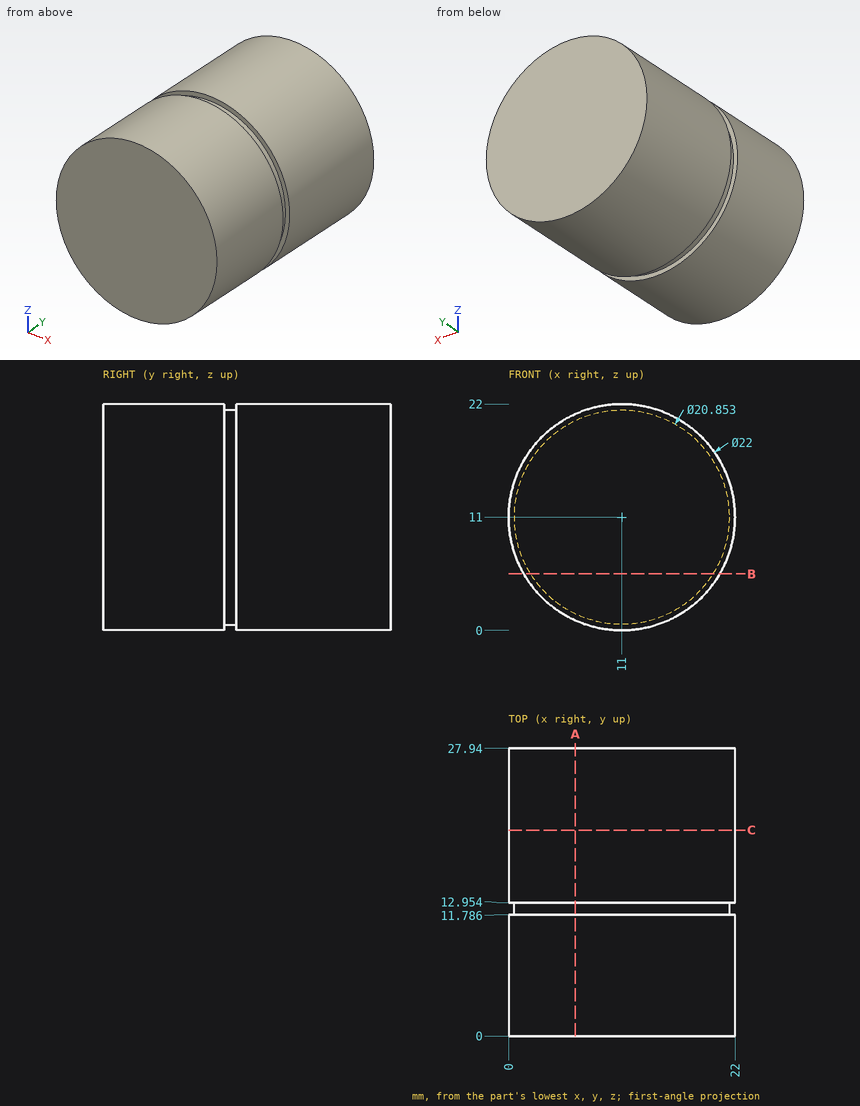
Design review of the part shown in the three views and the two pictorial views. Dimensions are in mm from the part's minimum x, y and z. Give positions to 0.01 mm unless a question says otherwise; leave off trailing zeros. Loops run counter-clockwise (first coordinate to the right, second up) from the corner with the lowest first, then second, coordinate; pieces in that order, holes last. Notation, with made-up numbers: (0, 85.5) -> (51, 85.5) arc R28 cw to (51, 116.5) -> close; hole circle Ø10 at (10.25, 22.25). An arc over 180 degrees is marked (long way). Answer as a JSON object with one key per item and string values. Group by question number.
Q1. Take a section at C-C (y = 20). Write out the cut boundary in (x, z).
Q2. Insertion check: pin 1 (8 mm diameter, centred on y = 23, z = 3.5, fed in from +X); pin 2 (12 mm diameter, centred on y = 13, z = 3, fed in from -X); pin 3 (2 mm diameter, centred on x = 16, y = 20.5, fed in from +Z). Each pin has a flat end and moves straight along its axis. Give the tip position at first contact, or say it passes through.
Q3. Wall thickness on line 1 along X through (y, z) = (11, 7.5); line 2 along X through (y, z) = (10.75, 15); line 3 along Z through (x, y) = (13.5, 18): over which ranges is each line inside the solid? List them lowest first.
Q4. Take a section at A-A (x = 6.5). Write out the cut boundary in (y, z) (1 decimal).
Q5. Take a section at B-B (z = 5.5). Write out the cut boundary in (x, y) (1 decimal), plus the area to 3 significant figures.
Answer below:
{
 "1": {"outline": "circle Ø22 at (11, 11)"},
 "2": {"pin 1": "stops at x = 21.43", "pin 2": "stops at x = 0.18", "pin 3": "stops at z = 21.25"},
 "3": {"line 1": "x = 0.57 to 21.43", "line 2": "x = 0.75 to 21.25", "line 3": "z = 0.29 to 21.71"},
 "4": {"outline": "(0, 1) -> (11.8, 1) -> (11.8, 1.6) -> (13, 1.6) -> (13, 1) -> (27.9, 1) -> (27.9, 21) -> (13, 21) -> (13, 20.4) -> (11.8, 20.4) -> (11.8, 21) -> (0, 21) -> close"},
 "5": {"outline": "(1.5, 0) -> (20.5, 0) -> (20.5, 11.8) -> (19.9, 11.8) -> (19.9, 13) -> (20.5, 13) -> (20.5, 27.9) -> (1.5, 27.9) -> (1.5, 13) -> (2.1, 13) -> (2.1, 11.8) -> (1.5, 11.8) -> close", "area": "531 mm2"}
}
